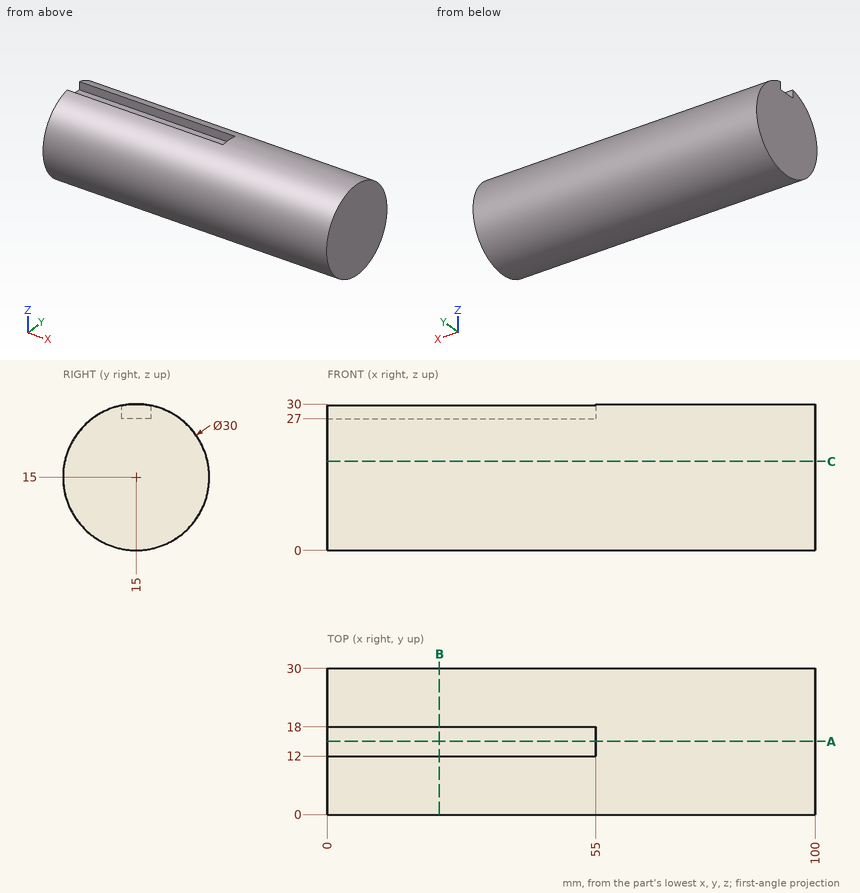
The figure shows three views and two pictorial views of one solid part (mm, origin at its lowest corner). Answer the questions. Coordinates: 2 decimals unless noted, no trailing zeros. Write each loop counter-clockwise with the first axis right and the second up, starting at its lowest first coordinate (ties: lowest second). Pieces come first, ordered by that corner, then holes. Notation, with made-up numbers: (43, 19.5) -> (47, 19.5) arc R19 cw to (47, 40.5) -> close; hole circle Ø8 at (-38.5, 72.5). An arc over 180 degrees is marked (long way). Return JSON: item names as keys, results as strings.
1. Find the intervals of material crossed by line 1 along Y through (x, z) = (7.5, 14.5); line 2 along Y through (x, z) = (23.5, 25); line 3 along Z through (x, y) = (14, 23.75), in increasing order. Write a range as from..to.
Found:
{"line 1": "0.01..29.99", "line 2": "3.82..26.18", "line 3": "2.82..27.18"}
2. A cutting plane is placed at A-A (y = 15). Determine the outline of the cut face in (x, z).
Found:
{"outline": "(0, 0) -> (100, 0) -> (100, 30) -> (55, 30) -> (55, 27) -> (0, 27) -> close"}
3. Each of these flat-tipped pins is pushed along its axis until it touches: P1, Ø1.5, axis at y = 16, z = 29, coming from the -X side; P2, Ø8, axis at x = 45.5, y = 7, coming from the +Z side; P3, Ø4, axis at x = 26.5, z = 7.5, coming from the +Y side. Where does it stop, or does it pass through?
Found:
{"P1": "x = 55", "P2": "z = 29.46", "P3": "y = 28.96"}
4. A cutting plane is placed at C-C (z = 18.25). Determine the outline of the cut face in (x, y).
Found:
{"outline": "(0, 0.36) -> (100, 0.36) -> (100, 29.64) -> (0, 29.64) -> close"}
5. A cutting plane is placed at B-B (x = 23). Determine the outline of the cut face in (y, z), and give its area (3 significant figures).
Found:
{"outline": "(12, 27) -> (12, 29.7) arc R15 ccw (long way) to (18, 29.7) -> (18, 27) -> close", "area": "689 mm2"}
